Could you check a few things on this model? Use its own coordinates, in mm. A direction names the side the tool comes from. Round coordinates to 2 decimals unless told otherwise and drop trailing zeros. Write each question's results on one line, items separated by ' | '.
from build123d import *

# Parameters (mm, degrees)
SKETCH1_W          = 300
SKETCH1_H          = 200
SKETCH2_W          = 320
SKETCH2_H          = 220
FILLET1_R          = 10
CUT_EXTRUDE1_DEPTH = 250
CUT_EXTRUDE3_DEPTH = 0.5
CUT_EXTRUDE4_DEPTH = 0.5


with BuildPart() as part:
    # Sketch1 → Loft1 section 0
    with BuildSketch(Plane(origin=(0, 0, 0), x_dir=(1, 0, 0), z_dir=(0, 1, 0))):
        Rectangle(SKETCH1_W, SKETCH1_H)
    # Sketch2 → Loft1 section 1
    with BuildSketch(Plane(origin=(0, 270, 0), x_dir=(1, 0, 0), z_dir=(0, 1, 0))):
        Rectangle(SKETCH2_W, SKETCH2_H)
    loft()

    # Fillet1
    fillet1_edges = [part.edges().sort_by_distance(p)[0] for p in [
        (155, 135, -105),
        (155, 135, 105),
        (-155, 135, 105),
        (-155, 135, -105),
    ]]
    fillet(fillet1_edges, radius=FILLET1_R)

    # Sketch3 → Cut-Extrude1 (cut)
    with BuildSketch(Plane(origin=(0, 270, 0), x_dir=(1, 0, 0), z_dir=(0, 1, 0))):
        with BuildLine():
            Line((-140, 100), (140, 100))
            ThreePointArc((140, 100), (147.071067812, 97.071067812), (150, 90))
            Line((150, 90), (150, -90))
            ThreePointArc((150, -90), (147.071067812, -97.071067812), (140, -100))
            Line((140, -100), (-140, -100))
            ThreePointArc((-140, -100), (-147.071067812, -97.071067812), (-150, -90))
            Line((-150, -90), (-150, 90))
            ThreePointArc((-150, 90), (-147.071067812, 97.071067812), (-140, 100))
        make_face()
    extrude(amount=-CUT_EXTRUDE1_DEPTH, mode=Mode.SUBTRACT)

    # Sketch4 → Cut-Extrude3 (cut)
    with BuildSketch(Plane(origin=(0, -3.698630137, 99.863013699), x_dir=(1, 0, 0), z_dir=(0, -0.037011661, 0.999314834))):
        with BuildLine():
            Line((-90.72593498, 3.701166051), (-72.75263326, 209.136944765))
            ThreePointArc((-72.75263326, 209.136944765), (-71.149610808, 212.387552735), (-67.77165977, 213.701166051))
            Line((-67.77165977, 213.701166051), (60.703357415, 213.701166051))
            ThreePointArc((60.703357415, 213.701166051), (64.015057291, 212.447183126), (65.665631129, 209.314223623))
            Line((65.665631129, 209.314223623), (90.668274157, 6.935256238))
            Line((90.668274157, 6.935256238), (91.067825571, 3.701166051))
            Line((91.067825571, 3.701166051), (-90.72593498, 3.701166051))
        make_face()
    cut_extrude3 = extrude(amount=-CUT_EXTRUDE3_DEPTH, mode=Mode.SUBTRACT)

    # Mirror1: Cut-Extrude3 across plane
    add(cut_extrude3.mirror(Plane.XY), mode=Mode.SUBTRACT)

    # Sketch5 → Cut-Extrude4 (cut)
    with BuildSketch(Plane(origin=(149.794520548, -5.547945205, 0), x_dir=(0, 0, -1), z_dir=(0.999314834, -0.037011661, 0))):
        with BuildLine():
            Line((-62.157161102, 5.551749076), (-44.583177002, 206.423306504))
            ThreePointArc((-44.583177002, 206.423306504), (-41.377132097, 212.924522445), (-34.621230021, 215.551749076))
            Line((-34.621230021, 215.551749076), (34.621230021, 215.551749076))
            ThreePointArc((34.621230021, 215.551749076), (41.377132097, 212.924522445), (44.583177002, 206.423306504))
            Line((44.583177002, 206.423306504), (62.157161102, 5.551749076))
            Line((62.157161102, 5.551749076), (-62.157161102, 5.551749076))
        make_face()
    cut_extrude4 = extrude(amount=-CUT_EXTRUDE4_DEPTH, mode=Mode.SUBTRACT)

    # Mirror2: Cut-Extrude4 across plane
    add(cut_extrude4.mirror(Plane(origin=(0, 0, 0), x_dir=(0, 0, 1), z_dir=(1, 0, 0))), mode=Mode.SUBTRACT)


solid = part.part
1) For faces 1 (the flat face through (2, 20, -1)), 2 (the cylindrical face through (-157.43, 207.31, -41.3)), 3 (the flat face through (-3, 0, -1)), which set-ups out of +Z, -Z, +X, -X, +Y, -Y let a thin tool reach every point of the face, with its end or its side?
Model answer:
face 1: +Y | face 2: -Y | face 3: +Z, -Z, +X, -X, -Y
2) I'm going to push flat-ended pins straight in: pin 1 (1.5 mm diameter, centred on y = 31.5, z = -47.5, fed in from +X); pin 2 (1.5 mm diameter, centred on x = -95, z = 82, fed in from +Y); pin 3 (3 mm diameter, centred on y = 194, z = 29, fed in from -X). Where does each tip first touch, or does it pass through?
Model answer:
pin 1: stops at x = 150.69 | pin 2: stops at y = 20 | pin 3: stops at x = -156.74
3) If we mould it in two halves opening along X, with no side actions, what happens to faces 4 (the flat face through (-15, 270, 105)), 5 (the flat face through (153.44, 106.42, -0.87)), 6 (the flat face through (1.44, 106.42, -103.44))? For each: released by +X, released by -X, zero draft, split by the parting line, or undercut.
Model answer:
face 4: zero draft | face 5: released by +X | face 6: undercut
4) I need wall thicknesses on line 1 (X direction, y = 211, z = 62.5); line 2 (Y direction, x = 43.5, z = 85); line 3 (Z direction, x = -113, y = 206.5). Which ranges of each line are inside material? Lowest first, please.
Model answer:
line 1: x = -157.81 to -150, 150 to 157.81 | line 2: y = 0 to 20 | line 3: z = -107.65 to -100, 100 to 107.65
